Verification items for the finished model (mm, model axes). Face numbers are marked on the shaded views. A direction names the side the tool comes from. Round coordinates to 2 decimals unless told otherwise and drop trailing zeros. Loops run counter-clockwise (first coordinate to the right, second up) from the corner with the lowest first, then second, coordinate; pieces in that order, holes last. Notation, with made-up numbers: (76, -26.5) -> (102, -26.5) arc R22 cw to (102, 8.5) -> close; hole circle Ø2 at (-13, -26.5). An arc over 180 degrees is marked (long way). Write item = value, one per line. Start each with the question number.
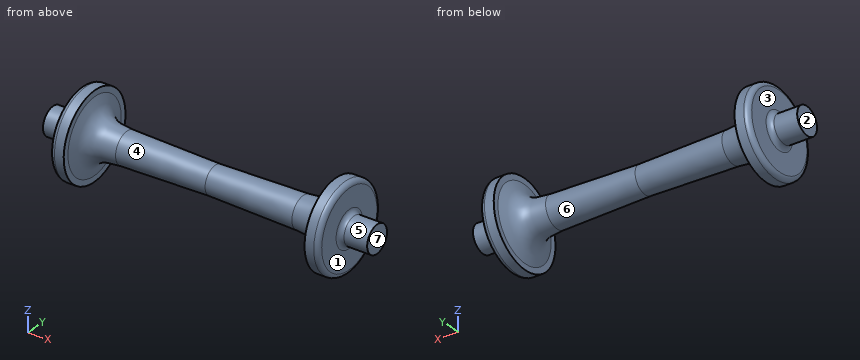
```python
from build123d import *


with BuildPart() as f1:
    # F0 (on Front) → F1 (revolve)
    with BuildSketch(Plane.XZ):
        with BuildLine():
            Line((-24.9903301983, 21.7737406916), (-113.2452650991, 19.8959766657))
            Line((-113.2452650991, 19.8959766657), (-113.2452650991, 4.8959766657))
            Line((-113.2452650991, 4.8959766657), (61.7547349009, 4.8959766657))
            Line((61.7547349009, 4.8959766657), (61.7547349009, 19.8959766657))
            Line((61.7547349009, 19.8959766657), (36.7547349009, 19.8959766657))
            ThreePointArc((36.7547349009, 19.8959766657), (33.2192009949, 21.3604427598), (31.7547349009, 24.8959766657))
            Line((31.7547349009, 24.8959766657), (31.7547349009, 46.6154164807))
            ThreePointArc((31.7547349009, 46.6154164807), (30.2902688068, 50.1509503867), (26.7547349009, 51.6154164807))
            Line((26.7547349009, 51.6154164807), (16.7547349009, 51.6154164807))
            Line((16.7547349009, 51.6154164807), (16.7547349009, 45.2127791941))
            add(Edge.make_bspline(
                [(16.7547349009, 45.2127791941), (14.6425744881, 38.1953757962), (10.3697433231, 23.9993991291), (-8.0631348251, 22.2263150664), (-18.0584447884, 21.9212275723)],
                knots=[0, 0, 0, 0, 0.4430583211, 0.8962924364, 0.8962924364, 0.8962924364, 0.8962924364], degree=3))
            add(Edge.make_bspline(
                [(-18.0584447884, 21.9212275723), (-20.3455392693, 21.8514184391), (-22.6679347338, 21.8125795654), (-24.9903301983, 21.7737406916)],
                knots=[0.8962924364, 0.8962924364, 0.8962924364, 0.8962924364, 1, 1, 1, 1], degree=3))
        make_face()
        with BuildLine():
            Line((-18.0584447884, 21.9212275723), (-24.9903301983, 21.7737406916))
            add(Edge.make_bspline(
                [(-18.0584447884, 21.9212275723), (-20.3455392693, 21.8514184391), (-22.6679347338, 21.8125795654), (-24.9903301983, 21.7737406916)],
                knots=[0.8962924364, 0.8962924364, 0.8962924364, 0.8962924364, 1, 1, 1, 1], degree=3))
        make_face()
    revolve(axis=Axis((-25.7452650991, 0, 4.8959766657), (1, 0, 0)))

    # F2: F1 across face


with BuildPart() as f1_1:
    add(f1.part)
    add(f1.part.mirror(Plane(origin=(-113.2452650991, 0, 4.8959766657), x_dir=(0, -1, 0), z_dir=(-1, 0, 0))))


solid = f1_1.part
```
(1) Section check B-B on x = -41. Enter the section's corners in (y, z).
(2) Scan lines: line 1 (X direction, y = -38, z = 15); line 2 (X direction, y = 24.5, z = -22); line 3 (Y direction, x = -185.5, z = 1). Record each from-to range of solid material in increasing order. Write a range as [from, to].
(3) Draft check along X on the marked faces 4, 5, 6 and 7. Enter one of: +X half, -X half, draft (parallel to the pull), parting line (faces both ways), or undercut.
(4) Section check A-A on x = -144.5. Enter the section's corners in (y, z) (3 decimals).
(5) Access from +Z, -Z, +X, -X, +Y, -Y to the whole of each face (thin tool, end or side, straight path). Record for the marked faces 1, 2 and 3.
(6) Depth check by flat-ended pin: pin 1 Ø3 at (x, y) = (-243, -14) entering from +Z; pin 2 Ø8 at (x, y) = (-206.5, 12) entering from +Z; pin 3 Ø2 at (y, z) = (-35, -13) entering from -X. Enter the tip coordinate at first touch or a pass-through.
Computed values:
q1.outline = circle Ø33.07 at (0, 4.9)
q2.line_1 = [-258.25, -242.94], [16.45, 31.75]
q2.line_2 = [-258.25, -242.03], [15.54, 31.75]
q2.line_3 = [-16.07, 16.07]
q3.face_4 = undercut
q3.face_5 = draft
q3.face_6 = undercut
q3.face_7 = +X half
q4.outline = circle Ø31.33 at (0, 4.896)
q5.face_1 = +X
q5.face_2 = +Z, -Z, -X, +Y, -Y
q5.face_3 = -X
q6.pin_1 = 49.91
q6.pin_2 = 19.88
q6.pin_3 = -258.25
